Geometry: final body of the model. Coordinates: model frame, mm. A direction names the side the tool comes from. Coordinates: 2 decimals unless noted, no trailing zeros. Order: outer loops, then holes, each group sorted by start corner. A loop starts at its lowest first (then second) coordinate and runs counter-clockwise, first axis right, second up. Notation, with made-up numbers: M 2.5,50 L 43.5,50 A23 ccw 43.5,58 Z; hole C 42,-17 d1. An arc over 180 degrees is marked long. Write item = value, one per line.
from build123d import *

# Parameters (mm, degrees)
ESBO_O1_W                  = 98
ESBO_O1_H                  = 98
RESSALTO_EXTRUS_O1_DEPTH   = 25
CORTE_EXTRUS_O4_DEPTH      = 74.668174947
CORTE_EXTRUS_O4_DEPTH_BACK = 74.668174947
CORTE_EXTRUS_O10_START     = 49
CORTE_EXTRUS_O10_DEPTH     = 20
CORTE_EXTRUS_O11_START     = -29
CORTE_EXTRUS_O11_DEPTH     = 20


with BuildPart() as part:
    # Esboço1 → Ressalto-extrusão1 (new, symmetric)
    with BuildSketch(Plane(origin=(0, 0, 0), x_dir=(1, 0, 0), z_dir=(0, 1, 0))):
        Rectangle(ESBO_O1_W, ESBO_O1_H)
    extrude(amount=RESSALTO_EXTRUS_O1_DEPTH, both=True)

    # Esboço2 → Corte-extrusão4 (cut, two sides: drawn at the far end of the back side and taken through both)
    with BuildSketch(Plane(origin=(0, 0, 0), x_dir=(0, 0, -1), z_dir=(1, 0, 0)).offset(-CORTE_EXTRUS_O4_DEPTH_BACK)):
        Polygon((-49, 25), (-49, -25), (-41, -20.381197846), (-14.799153207, 25), align=None)
    extrude(amount=CORTE_EXTRUS_O4_DEPTH + CORTE_EXTRUS_O4_DEPTH_BACK, mode=Mode.SUBTRACT)

    # Esboço7 → Corte-extrusão10 (cut)
    with BuildSketch(Plane(origin=(0, 0, 0), x_dir=(0, 0, -1), z_dir=(1, 0, 0)).offset(CORTE_EXTRUS_O10_START)):
        with BuildLine():
            ThreePointArc((33, -25), (44.313708499, -20.313708499), (49, -9))
            Line((49, -9), (33, -9))
            Line((33, -9), (33, -25))
        make_face()
        with BuildLine():
            ThreePointArc((33, 7), (44.313708499, 2.313708499), (49, -9))
            Line((49, -9), (49, 7))
            Line((49, 7), (33, 7))
        make_face()
        with BuildLine():
            Line((33, -9), (49, -9))
            ThreePointArc((49, -9), (44.313708499, 2.313708499), (33, 7))
            Line((33, 7), (33, -9))
        make_face()
        with BuildLine():
            Line((49, -25), (49, -9))
            ThreePointArc((49, -9), (44.313708499, -20.313708499), (33, -25))
            Line((33, -25), (49, -25))
        make_face()
        with BuildLine():
            Line((33, -25), (33, -9))
            Line((33, -9), (17, -9))
            ThreePointArc((17, -9), (21.686291501, -20.313708499), (33, -25))
        make_face()
        with BuildLine():
            Line((17, -9), (33, -9))
            Line((33, -9), (33, 7))
            ThreePointArc((33, 7), (21.686291501, 2.313708499), (17, -9))
        make_face()
        with BuildLine():
            Line((17, -25), (33, -25))
            ThreePointArc((33, -25), (21.686291501, -20.313708499), (17, -9))
            Line((17, -9), (17, -25))
        make_face()
    extrude(amount=-CORTE_EXTRUS_O10_DEPTH, mode=Mode.SUBTRACT)

    # Esboço9 → Corte-extrusão11 (cut)
    with BuildSketch(Plane(origin=(0, 0, 0), x_dir=(0, 0, -1), z_dir=(1, 0, 0)).offset(CORTE_EXTRUS_O11_START)):
        with BuildLine():
            Line((33, -25), (49, -25))
            Line((49, -25), (49, -9))
            ThreePointArc((49, -9), (44.313708499, -20.313708499), (33, -25))
        make_face()
        with BuildLine():
            ThreePointArc((17, -9), (21.686291501, -20.313708499), (33, -25))
            Line((33, -25), (33, -9))
            Line((33, -9), (17, -9))
        make_face()
        with BuildLine():
            Line((17, -25), (33, -25))
            ThreePointArc((33, -25), (21.686291501, -20.313708499), (17, -9))
            Line((17, -9), (17, -25))
        make_face()
        with BuildLine():
            Line((33, -9), (33, -25))
            ThreePointArc((33, -25), (44.313708499, -20.313708499), (49, -9))
            Line((49, -9), (33, -9))
        make_face()
        with BuildLine():
            ThreePointArc((33, 7), (44.313708499, 2.313708499), (49, -9))
            Line((49, -9), (49, 7))
            Line((49, 7), (33, 7))
        make_face()
        with BuildLine():
            Line((33, -9), (49, -9))
            ThreePointArc((49, -9), (44.313708499, 2.313708499), (33, 7))
            Line((33, 7), (33, -9))
        make_face()
        with BuildLine():
            Line((17, -9), (33, -9))
            Line((33, -9), (33, 7))
            ThreePointArc((33, 7), (21.686291501, 2.313708499), (17, -9))
        make_face()
    extrude(amount=-CORTE_EXTRUS_O11_DEPTH, mode=Mode.SUBTRACT)


solid = part.part
1) Mould query, pull axis X, two halves, no side actions, for faces 4 (the face through (49, 0, 1)), 5 (the face through (-49, 0, 1)), 6 (the face through (-1, 25, -18)). Classes: pulls with the +X half, pulls with the -X half, needs draft (parallel to the pull), parting line crosses it, or undercut.
Numbers:
face_4 = pulls with the +X half
face_5 = pulls with the -X half
face_6 = needs draft
2) Section D-D, the plane x = 21. Return loops of the section in (y, z), and give its area (3 significant figures).
Numbers:
outline = M -25,-49 L 25,-49 L 25,14.8 L -20.38,41 L -25,49 Z
area = 3,920 mm²
3) Set-up query: faces 1 (the face through (-39, -17, -17)), 2 (the face through (39, 7, -41)), 3 (the face through (-1, 6, -49)). Return all of +Z, -Z, +X, -X, +Y, -Y with unobstructed straight access to the full face (end or side cutting, diameter ignored); none if empty.
Numbers:
face_1 = -Z, -X, -Y
face_2 = -Z, +X, -Y
face_3 = -Z, +X, -X, +Y, -Y
4) Section C-C, the plane y = 13. Return loops of the section in (x, z).
Numbers:
outline = M -49,-49 L 49,-49 L 49,21.73 L -49,21.73 Z
5) Pin query (flat end, axial travel): pin 1 (9.5 mm diameter, centred on y = -15.5, z = -38, fed in from +X); pin 2 (13 mm diameter, centred on x = -35, z = -38.5, fed in from -Y); pin 3 (8 mm diameter, centred on x = 40, z = -40, fed in from -Y); pin 4 (13 mm diameter, centred on x = -36, y = -13, fed in from -Z). Return the tip coordinate at first contact, or that it passes through.
Numbers:
pin_1 = 29
pin_2 = -25
pin_3 = 7
pin_4 = -17.2
6) Section A-A, the plane z = -38.5. Return loops of the section in (x, y), and give its area (3 significant figures).
Numbers:
outline = M -49,7 L -29,7 L -29,-25 L 29,-25 L 29,7 L 49,7 L 49,25 L -49,25 Z
area = 3,620 mm²
7) Section B-B, the plane x = 43. Return loops of the section in (y, z), and give its area (3 significant figures).
Numbers:
outline = M -25,-17 L -9,-17 A16 cw 7,-33 L 7,-49 L 25,-49 L 25,14.8 L -20.38,41 L -25,49 Z
area = 2,950 mm²
8) Line query: L1, parallel to Y at x = -38.5, z = -43.5; L2, parallel to X at y = -23, z = -21; L3, parallel to Z at x = 11.5, y = -4.5. Output: solid intervals per line, ascending.
Numbers:
L1 = 7 to 25
L2 = -29 to 29
L3 = -49 to 31.83
